Can you work these out from the model? Positions are in its coordinate system, mm. A direction names the side the tool comes from. Give positions to 0.01 mm unless a question says otherwise; leave off trailing zeros. Loops run counter-clockwise (first coordinate to the right, second up) from the corner with the lowest first, then second, coordinate; pieces in that order, holes last. Notation, with made-up numbers: (36, 21.5) -> (85, 21.5) arc R28 ccw to (85, 41.5) -> close; hole circle Ø8 at (4.5, 20.5). An arc over 180 degrees is marked (long way). One line per question, with ' | ' between items.
Autodesk Inventor part; units mm, degrees
ref_plane "YZ Plane" through (0, 0, 0) normal (1, 0, 0) x (0, 1, 0)
ref_plane "XZ Plane" through (0, 0, 0) normal (0, 1, 0) x (-1, 0, 0)
ref_plane "XY Plane" through (0, 0, 0) normal (0, 0, 1) x (1, 0, 0)
sketch "Sketch1" plane through (0, 0, 0) normal (0, 0, 1) x (1, 0, 0)
  line L0 (0, 0) -> (0, 15)
  line L1 (0, 15) -> (-2.7, 15)
  line L2 (-2.7, 15) -> (-2.7, 12)
  line L3 (-2.7, 12) -> (-1.5, 12)
  line L4 (-1.5, 12) -> (-1.5, 0)
  line L5 (-1.5, 0) -> (0, 0)
  dimension "d0" = 12
  dimension "d1" = 3
  dimension "d2" = 1.5
  dimension "d3" = 2.7
revolve "Revolution1" add sketch "Sketch1" angle 360 about axis through (0, 0, 0) along (0, 1, 0)
sketch "Sketch2" plane through (0, 15, 0) normal (0, 1, 0) x (1, 0, 0)
  line L0 (-0.7217, -1.25) -> (-1.4434, 0)
  line L1 (-1.4434, 0) -> (-0.7217, 1.25)
  line L2 (-0.7217, 1.25) -> (0.7217, 1.25)
  line L3 (0.7217, 1.25) -> (1.4434, 0)
  line L4 (1.4434, 0) -> (0.7217, -1.25)
  line L5 (0.7217, -1.25) -> (-0.7217, -1.25)
  point P0 (0, 0)
  point P1 (0, 0)
  dimension "d5" = 2.5
extrude "Extrusion1" cut sketch "Sketch2" against normal blind 2
fillet "Fillet1" radius 0.3 6 edges at (0, 15, -1.25) (1.0825, 15, -0.625) (1.0825, 15, 0.625) (0, 15, 1.25) (-1.0825, 15, 0.625) (-1.0825, 15, -0.625)
fillet "Fillet2" radius 0.3 1 edges at (2.7, 15, 0)
thread "Thread1"
properties part number "Screw_M4X12_SS_HEX" material "Stainless Steel"
Q1. If I drill on probe 1 along Y at (x, z) = (0.1, 0.6); probe 2 along Y at (x, z) = (0.55, -2.35); probe 3 along Z at (x, y) = (0.1, 10), over which ranges is the centre line in solid material (lowest first)? Write a range as from..to.
Entries:
probe 1: 0..13 | probe 2: 12..15 | probe 3: -1.5..1.5
Q2. If we section it at A-A (x = 0): Write out the boundary of the cut face in (y, z), plus the area to 3 significant figures.
Entries:
outline: (0, -1.5) -> (12, -1.5) -> (12, -2.7) -> (14.7, -2.7) arc R0.3 ccw to (15, -2.4) -> (15, -1.55) arc R0.3 ccw to (14.7, -1.25) -> (13, -1.25) -> (13, 1.25) -> (14.7, 1.25) arc R0.3 ccw to (15, 1.55) -> (15, 2.4) arc R0.3 ccw to (14.7, 2.7) -> (12, 2.7) -> (12, 1.5) -> (0, 1.5) -> close | area: 47.1 mm²
Q3. For pin 1 Ø2 at (y, z) = (8.5, 0) entering from -X; pin 2 Ø0.8 at (x, z) = (-0.5, 0) entering from +Y, each with a flat end and sliding along its axis, tell me the tip position at first contact or that it passes through.
Entries:
pin 1: x = -1.5 | pin 2: y = 13
Q4. If we mould it in two halves opening along X, with no side actions, what happens to faces 1 (the face through (0, 14, 1.25)), 2 (the face through (1.5, 5.92, -0.07)), 3 (the face through (0, 14, -1.25)), 4 (the face through (0, 0, 0))? For each: pulls with the +X half, pulls with the -X half, needs draft (parallel to the pull), parting line crosses it, or undercut.
Entries:
face 1: undercut | face 2: parting line crosses it | face 3: undercut | face 4: needs draft
Q5. On a 3-axis mill with a long thin cutter (end or side, diameter ignored), from which of +Z, -Z, +X, -X, +Y, -Y can I reach the whole of each face in a straight line? I mean faces 5 (the face through (-1.2, 12, -1.2)), 6 (the face through (0.585, 13.331, 2.636)), 7 (the face through (0, 13, 0)). Say none if no direction works.
Entries:
face 5: -Y | face 6: +Y, -Y | face 7: +Y
Q6. If we section it at B-B (y = 7.25): Write out the boundary of the cut face in (x, z), plus the area to 3 significant figures.
Entries:
outline: circle Ø3 at (0, 0) | area: 7.07 mm²
